Could you check a few things on this model? Use its own coordinates, in mm. A direction names the side the tool comes from. Round coordinates to 2 decimals unless told otherwise and drop trailing zeros. Loops run counter-clockwise (first coordinate to the right, second up) from the corner with the lowest first, then second, coordinate; pieces in that order, holes last. Notation, with made-up numbers: (-27.5, 27.25) - (30.5, 27.25) arc R28 ccw to (30.5, 66.25) - close; hole circle Ø1 at (-21, 36.25). An arc over 180 degrees is marked (long way). Use one line per item in the form item = value.
Autodesk Inventor part; units mm, degrees
ref_plane "YZ Plane" through (0, 0, 0) normal (1, 0, 0) x (0, 1, 0)
ref_plane "XZ Plane" through (0, 0, 0) normal (0, 1, 0) x (-1, 0, 0)
ref_plane "XY Plane" through (0, 0, 0) normal (0, 0, 1) x (1, 0, 0)
sketch "Sketch1" plane through (0, 0, 0) normal (1, 0, 0) x (0, 1, 0)
  line L0 (0, 0) -> (0, 25)
  line L1 (0, 25) -> (48.2963, 37.941)
  line L2 (48.2963, 37.941) -> (48.2963, 42.941)
  line L3 (48.2963, 42.941) -> (46.2963, 42.941)
  line L4 (0, 25) -> (0, 28)
  line L5 (0, 28) -> (46.2963, 40.4051)
  line L6 (0, 28) -> (-3, 28)
  line L7 (-3, 28) -> (-3, 0)
  line L8 (-3, 0) -> (0, 0)
  line L9 (0, 0) -> (0, 28)
  line L10 (46.2963, 42.941) -> (46.2963, 40.4051)
  line L11 (0, 28) -> (0, 25)
  line L12 (0, 25) -> (48.2963, 37.941)
  line L13 (48.2963, 37.941) -> (48.2963, 42.941)
  line L14 (48.2963, 42.941) -> (46.2963, 42.941)
  line L15 (46.2963, 42.941) -> (46.2963, 40.4051)
  line L16 (46.2963, 40.4051) -> (0, 28)
  line L17 (0, 28) -> (0, 25)
  dimension "d0" = 25
  dimension "d1" = 50
  dimension "d2" = 105
  dimension "d3" = 5
  dimension "d4" = 2
  dimension "d5" = 3
  dimension "d6" = 105
  dimension "d7" = 3
sketch "Sketch2" plane through (0, 0, 0) normal (1, 0, 0) x (0, 1, 0)
  line L0 (0, 0) -> (3.3899, 0)
revolve "Revolution1" add sketch "Sketch1" angle 360 about axis through (0, 0, 0) along (0, 1, 0)
fillet "Fillet1" radius 2 1 edges at (0, -3, -28)
properties part number "_3DPrint"
1. Please list where these lines run through material, in increasing order: line 1 along Y through (x, z) = (0, 0.5); line 2 along Z through (x, y) = (-23, 30); line 3 along X through (y, z) = (32.5, 13).
Solution:
line_1 = -3 to 0
line_2 = -27.74 to -23.72, 23.72 to 27.74
line_3 = -34.33 to -31.1, 31.1 to 34.33
2. For P1, Ø5, axis at y = 15.5, z = 12, coming from the -X side; P2, Ø10, axis at x = 33, y = 29.5, coming from the +Z side; P3, Ø5, axis at x = -22.5, y = 35.5, coming from the -Z side, each with a flat end and sliding along its axis, tell me the tip position at first contact or that it passes through.
Solution:
P1 = -30.98
P2 = 22.83
P3 = -31.92
3. On a 3-axis mill with a long thin cutter (end or side, diameter ignored), from which of +Z, -Z, +X, -X, +Y, -Y can I reach the whole of each face in a straight line? I mean faces 4 (the face through (-25, 46.296, 32)), 5 (the face through (0, -3, 0)). Say none if no direction works.
Solution:
face_4 = -Y
face_5 = +Z, -Z, +X, -X, -Y
4. If we section it at A-A, the plane x = 0: Write out the boundary of the cut face in (y, z).
Solution:
outline = (-3, -26) arc R2 ccw to (-1, -28) - (0, -28) - (46.3, -40.41) - (46.3, -42.94) - (48.3, -42.94) - (48.3, -37.94) - (0, -25) - (0, 25) - (48.3, 37.94) - (48.3, 42.94) - (46.3, 42.94) - (46.3, 40.41) - (0, 28) - (-1, 28) arc R2 ccw to (-3, 26) - close
5. If we section it at B-B, the plane z = 0: Write out the boundary of the cut face in (x, y), plus the area to 3 significant figures.
Solution:
outline = (-42.94, 46.3) - (-40.41, 46.3) - (-28, 0) - (-28, -1) arc R2 ccw to (-26, -3) - (26, -3) arc R2 ccw to (28, -1) - (28, 0) - (40.41, 46.3) - (42.94, 46.3) - (42.94, 48.3) - (37.94, 48.3) - (25, 0) - (-25, 0) - (-37.94, 48.3) - (-42.94, 48.3) - close
area = 465 mm^2
6. If we section it at D-D, the plane y = 15: Write out the boundary of the cut face in (x, z).
Solution:
outline = circle Ø64.04 at (0, 0); hole circle Ø58.04 at (0, 0)
7. If we section it at C-C, the plane y = 1.5: Write out the boundary of the cut face in (x, z).
Solution:
outline = circle Ø56.8 at (0, 0); hole circle Ø50.8 at (0, 0)
8. We'd pull the mould along Z, two halves only. Please class faces 1 (the face through (0, 0, 0)), 2 (the face through (-38, 48.296, 3)), 3 (the face through (10.724, -0.507, 25.865)): +Z half, -Z half, draft (parallel to the pull), parting line (faces both ways), or undercut.
Solution:
face_1 = undercut
face_2 = draft
face_3 = parting line
